```python
from build123d import *

# Parameters (mm, degrees)
EXTRUDE_1_DEPTH     = 16
SKETCH_3_R          = 1.475
CUT_EXTRUDE_1_DEPTH = 32.020154738
EXTRUDE_2_DEPTH     = 5
EXTRUDE_START       = 0.5
SKETCH_5_R          = 2.5
SKETCH_5_R_2        = 1.475
EXTRUDE_3_DEPTH     = 0.5
SKETCH_6_R          = 1.5
EXTRUDE_4_DEPTH     = 4


with BuildPart() as part:
    # Эскиз2 → Бобышка-Вытянуть1 (new body)
    with BuildSketch(Plane(origin=(0, 0, 0), x_dir=(1, 0, 0), z_dir=(0, 1, 0))):
        Polygon((-20, 5), (-5, 17.5), (0, 17.5), (0, 0), (-20, 0), align=None)
    extrude(amount=EXTRUDE_1_DEPTH)

    # Эскиз3 → Вырез-Вытянуть1 (cut, through all)
    with BuildSketch(Plane(origin=(0, 16, 0), x_dir=(1, 0, 0), z_dir=(0, 1, 0))):
        with Locations(Location((-2.5, 14.5, 0), (0, 0, 270))):
            Circle(SKETCH_3_R)
        with Locations(Location((-2.5, 3, 0), (0, 0, 270))):
            Circle(SKETCH_3_R)
    extrude(amount=-CUT_EXTRUDE_1_DEPTH, mode=Mode.SUBTRACT)

    # Эскиз4 → Бобышка-Вытянуть2 (add)
    with BuildSketch(Plane(origin=(0, 16, 0), x_dir=(1, 0, 0), z_dir=(0, 1, 0))):
        Polygon((-20, 4), (-20, 0), (-14, 0), (-14, 1.5), align=None)
    extrude(amount=EXTRUDE_2_DEPTH)

    # Эскиз5 → Бобышка-Вытянуть3 (add)
    with BuildSketch(Plane(origin=(0, 16, 0), x_dir=(1, 0, 0), z_dir=(0, 1, 0)).offset(EXTRUDE_START)):
        with Locations((-2.5, 14.5)):
            Circle(SKETCH_5_R)
        with Locations(Location((-2.5, 14.5, 0), (0, 0, 270))):
            Circle(SKETCH_5_R_2, mode=Mode.SUBTRACT)
    extrude(amount=-EXTRUDE_3_DEPTH)

    # Эскиз6 → Бобышка-Вытянуть4 (add)
    with BuildSketch(Plane(origin=(-1.538461538, 0, 3.692307692), x_dir=(-0.9230769230769231, 0, -0.3846153846153845), z_dir=(0.3846153846153845, 0, -0.9230769230769231))):
        with Locations(Location((16.75, 18.5, 0), (0, 0, 180))):
            Circle(SKETCH_6_R)
    extrude(amount=EXTRUDE_4_DEPTH)


solid = part.part
```
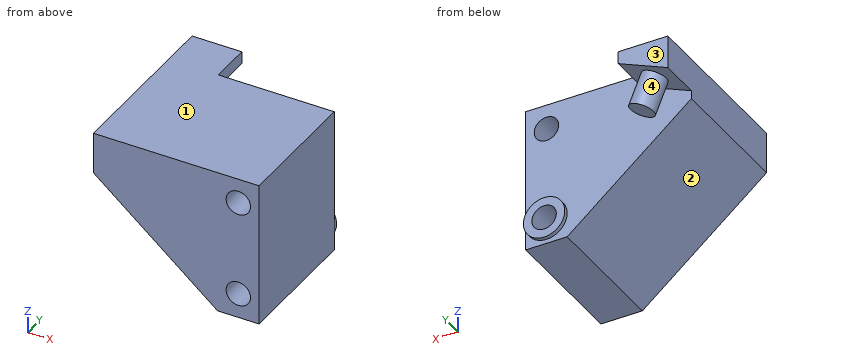
The listing builds one solid part. Answer for the finished solid, in the listing's coordinates (mm). Face numbers are marked on the shaded views. Coordinates: 2 decimals unless noted, no trailing zeros. Loops run counter-clockwise (first coordinate to the right, second up) from the corner with the lowest first, then second, coordinate; pieces in that order, holes last. Notation, with made-up numbers: M 42,-14 L 49,-14 A25 cw 49,9 Z; hole C 28.25,33.5 d4. An arc over 180 degrees is marked long. Answer as CSV lines item,"result". Start each with the question number.
(1) Find the intervals of material crossed by L1, parallel to X at y = 5.5, z = -3 (3 decimals); L2, parallel to Y at x = -14, z = -6.5; L3, parallel to X at y = 6.25, z = -14.5 (3 decimals), in increasing order. Write a range as [from, to].
(2) The part is cut by section C-C (z = -10.75). Give the vertices of the cut face in (x, y), and give its area (3 significant figures).
(3) The part is cut by section D-D (x = -7.25). Give the vertices of the cut face in (y, z) (3 decimals), and give its area (3 significant figures).
(4) Given pin 1 (2 mm diameter, centred on x = -7.5, y = 6, fed in from -Z); pin 2 (1.8 mm diameter, centred on x = -2.5, z = -14.5, fed in from +Y); pin 3 (0.8 mm diameter, centred on y = 19, z = -0.5, fed in from +X); pin 4 (4 mm diameter, centred on x = -1.5, z = -14.5, fed in from +Y), each flat-ended and moving along its own axis, determine where each tip first touches the part or whether it passes through.
(5) The part is cut by section B-B (y = 14). Give the vertices of the cut face in (x, z) (3 decimals), and give its area (3 significant figures).
(6) The part is cut by section A-A (x = -2.5). Give the vertices of the cut face in (y, z) (3 decimals).
(7) The mould has two halves that part along Z. Classify the marked faces 1, 2, 3 and 4: pulls with the +Z half, pulls with the -Z half, needs draft (parallel to the pull), parting line crosses it, or undercut.
Determined:
1,L1,"[-20, -3.975], [-1.025, 0]"
1,L2,"[0, 16]"
1,L3,"[-8.6, -3.975], [-1.025, 0]"
2,outline,"M -13.1,0 L 0,0 L 0,16 L -13.1,16 Z"
2,area,"210 mm2"
3,outline,"M 0,-15.625 L 16,-15.625 L 16,0 L 0,0 Z"
3,area,"250 mm2"
4,pin 1,"z = -16.25"
4,pin 2,"through"
4,pin 3,"x = -14"
4,pin 4,"y = 16.5"
5,outline,"M -20,-5 L -5,-17.5 L 0,-17.5 L 0,0 L -20,0 Z; hole C -2.5,-14.5 d2.95; hole C -2.5,-3 d2.95"
5,area,"243 mm2"
6,outline,"M 0,-17.5 L 16,-17.5 L 16,-17 L 16.5,-17 L 16.5,-15.975 L 0,-15.975 Z; M 0,-13.025 L 16.5,-13.025 L 16.5,-12 L 16,-12 L 16,-4.475 L 0,-4.475 Z; M 0,-1.525 L 16,-1.525 L 16,0 L 0,0 Z"
7,face 1,"pulls with the +Z half"
7,face 2,"pulls with the -Z half"
7,face 3,"needs draft"
7,face 4,"undercut"
